The listing builds one solid part. Answer for the finished solid, in the listing's coordinates (mm). Face numbers are marked on the shaded views. Round coordinates to 2 decimals unless told otherwise and drop trailing zeros. Order: outer loops, then holes, each group sorted by start corner. A loop starts at its lowest first (then second) coordinate and runs counter-clockwise, first axis right, second up. Notation, with made-up numbers: (-7.5, 38.25) - (20.5, 38.25) arc R16 cw to (20.5, 53.25) - close; hole circle Ø3 at (39, 79.5). An arc over 180 degrees is marked (long way). One line per item, written item: value. Start each with the question number.
1. Section C-C, the plane x = 0.65 is taken. Give the vertices of the cut face in (y, z).
2. Straight lines are drawn through the part: line 1 (X direction, y = 5.75, z = 0); line 2 (Z direction, x = 0.65, y = 2); line 3 (Z direction, x = 0.85, y = 3). For each, find the intervals that lie inside material, in ascending order.
3. Flat-ended cylindrical pins translate along their axes: P1, Ø1.5, axis at y = 6, z = 2, coming from the +X side; P2, Ø1, axis at x = 1, y = 6, coming from the +Z side. Find the tip coordinate at first contact, or state that the pin passes through.
4. Section D-D, the plane z = 2.3 is taken. Give the vertices of the cut face in (x, y).
5. Section A-A, the plane y = 0.75 is taken. Give the vertices of the cut face in (x, z), then the cut area to 3 significant figures.
6. Section B-B, the plane z = -0.2 is taken. Give the vertices of the cut face in (x, y), then the cut area to 3 significant figures.
7. For a pull along X with two mould halves and no side action, classify the marked faces 1, 2 and 3 as released by +X, released by -X, zero draft, split by the parting line, or undercut.
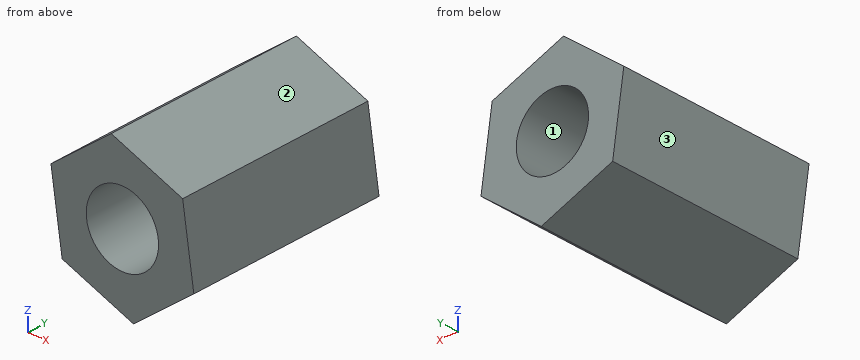
from build123d import *

# Parameters (mm, degrees)
SALIENTE_EXTRUIR1_DEPTH = 7
CROQUIS_CARA_R          = 1.25
CORTAR_EXTRUIR1_DEPTH   = 7


with BuildPart() as part:
    # Croquis base → Saliente-Extruir1 (new body)
    with BuildSketch(Plane(origin=(0, 0, 0), x_dir=(1, 0, 0), z_dir=(0, 1, 0))):
        Polygon((2.082277712, -1.648469855), (2.468755628, 0.979070469), (0.386477916, 2.627540324), (-2.082277712, 1.648469855), (-2.468755628, -0.979070469), (-0.386477916, -2.627540324), align=None)
    extrude(amount=SALIENTE_EXTRUIR1_DEPTH)

    # Croquis cara → Cortar-Extruir1 (cut)
    with BuildSketch(Plane(origin=(0, 7, 0), x_dir=(1, 0, 0), z_dir=(0, 1, 0))):
        with Locations(Location((0, 0, 0), (0, 0, 270))):
            Circle(CROQUIS_CARA_R)
    extrude(amount=-CORTAR_EXTRUIR1_DEPTH, mode=Mode.SUBTRACT)


solid = part.part
Answer list:
1. outline: (0, -2.42) - (7, -2.42) - (7, -1.07) - (0, -1.07) - close; (0, 1.07) - (7, 1.07) - (7, 2.22) - (0, 2.22) - close
2. line 1: x = -2.32 to -1.25, 1.25 to 2.32
2. line 2: z = -2.42 to -1.07, 1.07 to 2.22
2. line 3: z = -2.26 to -0.92, 0.92 to 2.14
3. P1: stops at x = 2.14
3. P2: stops at z = 2.28
4. outline: (-0.8, 0) - (0.44, 0) - (0.44, 7) - (-0.8, 7) - close
5. outline: (-2.47, 0.98) - (-2.08, -1.65) - (0.39, -2.63) - (2.47, -0.98) - (2.08, 1.65) - (-0.39, 2.63) - close; hole circle Ø2.5 at (0, 0)
5. area: 13.4 mm²
6. outline: (-2.3, 0) - (-1.23, 0) - (-1.23, 7) - (-2.3, 7) - close; (1.23, 0) - (2.35, 0) - (2.35, 7) - (1.23, 7) - close
6. area: 15.3 mm²
7. face 1: undercut
7. face 2: released by +X
7. face 3: released by -X
